Autodesk Inventor part; units mm, degrees
ref_plane "YZ Plane" through (0, 0, 0) normal (1, 0, 0) x (0, 1, 0)
ref_plane "XZ Plane" through (0, 0, 0) normal (0, 1, 0) x (-1, 0, 0)
ref_plane "XY Plane" through (0, 0, 0) normal (0, 0, 1) x (1, 0, 0)
sketch "草圖1" plane through (0, 0, 0) normal (0, 1, 0) x (-1, 0, 0)
  circle A0 centre (0, 0) radius 4
  dimension "d0" = 8
extrude "擠出1" add sketch "草圖1" along normal blind 5
sketch "草圖2" plane through (0, 0, 0) normal (0, -1, 0) x (1, 0, 0)
  circle A0 centre (0, 0) radius 2.5
  dimension "d3" = 5
extrude "擠出2" cut sketch "草圖2" against normal blind 3
sketch "草圖3" plane through (0, 5, 0) normal (0, 1, 0) x (1, 0, 0)
  circle A0 centre (0, 0) radius 2.5
  dimension "d6" = 5
extrude "擠出3" add sketch "草圖3" along normal blind 3
chamfer "倒角1" distance 1.5 angle 45 1 edges at (-2.5, 5, 0)
sketch "草圖4" plane through (0, 0, 0) normal (0, 0, 1) x (1, 0, 0)
  arc A0 (0, 7.3301) -> (0, 17.3301) centre (0, 12.3301) ccw
  line L0 (0, 12.3301) -> (0, 17.3301) construction
  line L1 (0, 12.3301) -> (0, 7.3301) construction
  line L2 (0, 17.3301) -> (0, 7.3301)
  line L3 (2.5, 8) -> (-2.5, 8)
  point P0 (0, 0)
  dimension "d12" = 5
  dimension "d13" = 180
  dimension "d14" = 90
  dimension "d15" = 2.5
revolve "迴轉1" add sketch "草圖4" angle 360 about axis through (0, 12.3301, 0) along (0, -1, 0)
fillet "圓角1" radius 4 1 edges at (-2.5, 8, 0)
sketch "草圖6" plane through (0, 0, 0) normal (0, -1, 0) x (1, 0, 0)
  circle A0 centre (0, 0) radius 2.5
  line L0 (-1, 2.2913) -> (1, 2.2913)
  line L1 (1, 2.2913) -> (1, 3.5913)
  line L2 (1, 3.5913) -> (-1, 3.5913)
  line L3 (-1, 3.5913) -> (-1, 2.2913)
  dimension "d20" = 2
  dimension "d21" = 1.3
extrude "擠出5" cut sketch "草圖6" against normal blind 3 contours A0 L3 L2 L1
fillet "圓角2" radius 2 1 edges at (-2.5, 6.4999, 0)
sketch "草圖5" plane through (0, 0, 0) normal (0, -1, 0) x (1, 0, 0)
  circle A0 centre (0, 0) radius 3.2143
  circle A1 centre (0, 0) radius 2.5
  circle A2 centre (0, 0) radius 4
properties part number "伸縮缸 球軸 球"
Check sheet for the modelled part. Datum: model origin and axes. Units: mm. Coordinates: 2 decimals unless noted, no trailing zeros. Order: outer loops, then holes, each group sorted by start corner. A loop starts at its lowest first (then second) coordinate and runs counter-clockwise, first axis right, second up. Notation, with made-up numbers: M 17.25,-28.75 L 41.25,-28.75 A34 cw 41.25,5.25 Z; hole C 77.5,45.25 d9. An arc over 180 degrees is marked long. One line per question, with ' | ' between items. Start each with the question number.
Item 1: Sectioned sample at A-A on y = 3.25. Record the cut outline in (x, z), and give its area (3 significant figures).
Item 2: Material ranges on line 1 (Z direction, x = 0, y = 2.25); line 2 (Y direction, x = -1.5, z = -3.5); line 3 (Z direction, x = -1.75, y = 10.5), recorded low to high.
Item 3: Mould release check, pull along Z, two halves, no side actions. Record for faces 1 (the cylindrical face through (0.867, 2.465, 3.905)), 2 (the flat face through (0, 0, -3)), 3 (the flat face through (1, 1, 3)): pulls with the +Z half, pulls with the -Z half, needs draft (parallel to the pull), parting line crosses it, or undercut.
Item 4: Sectioned sample at B-B on z = 4.25. Record the cut outline in (x, y), and give its area (3 significant figures).
Item 5: Gauge pin test, flat ends, axial feed: P1, Ø3, axis at y = 8, z = 3, coming from the +X side; P2, Ø1.6, axis at x = 0, y = 2, coming from the -Z side; P3, Ø1.5, axis at x = -1.5, z = -2, coming from the +Y side. Record the tip position at first contact, or that the pin passes through.
Answer below:
1) outline: C 0,0 d8 | area: 50.3 mm^2
2) line 1: z = -4 to -2.5, 3.59 to 4 | line 2: y = 0 to 5.19, 9.09 to 15.57 | line 3: z = -4.31 to 4.31
3) face 1: parting line crosses it | face 2: needs draft | face 3: undercut
4) outline: C 0,12.33 d5.27 | area: 21.8 mm^2
5) P1: stops at x = 3.29 | P2: stops at z = -4 | P3: stops at y = 17.01
